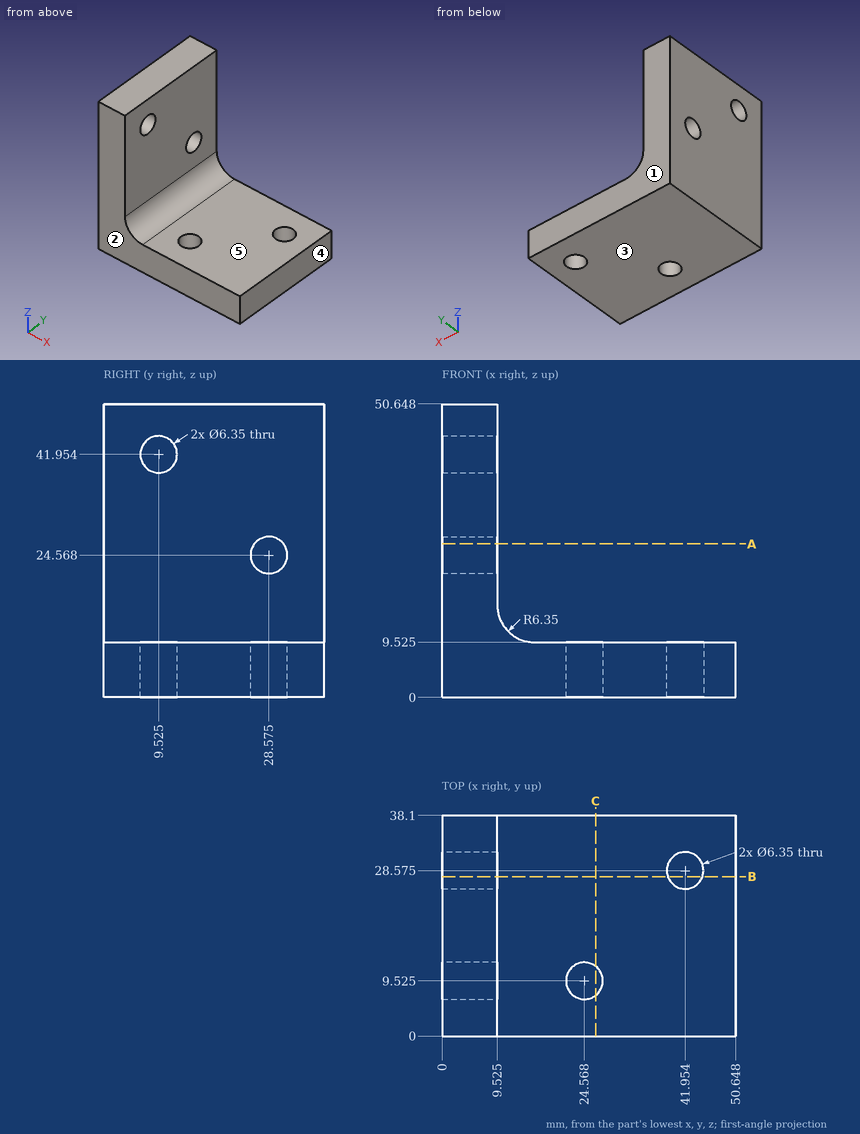
Source: three-view drawing plus pictorial views. Frame: mm from the lowest corner of the part. A direction names the side the tool comes from. Give positions to 0.01 mm unless a question says otherwise; leave off trailing zeros. Write each loop counter-clockwise with the first axis right and the second up, starting at its lowest first coordinate (ties: lowest second). Pieces come first, ordered by that corner, then holes. Notation, with made-up numbers: (-31.5, -10) - (-26.5, -10) arc R9 cw to (-26.5, 2) - close; hole circle Ø2 at (80, -12). An arc over 180 degrees is marked (long way). Write item = value, one per line. Start each with the question number.
1. Ray query, L1, parallel to X at y = 35.5, z = 43 (1 decimal); L2, parallel to Y at x = 5.5, z = 44.5 (1 decimal). Return the intervals inside material, ascending.
2. Section query B-B, the plane y = 27.5. Count the separate pieces of the cut face and the enclosed holes in it, then the cut area to 3 significant figures.
3. Section query A-A, the plane z = 26.5. Output: boundary loops of the cut face in (x, y) (1 decimal), then the cut area to 3 significant figures.
4. Access query for the marked faces 4 and 5. Directions: +Z, -Z, +X, -X, +Y, -Y. A direction counts if a zero-diameter tool reaches every point of the face in a straight line with its end or side. Return the directions, or none.
5. First-contact query: pin 1 Ø17.5 at (y, z) = (12, 40.5) entering from +X (3 decimals). Flat tip, straight axial feed; report the tip coordinate or a pass-through.
6. Section query C-C, the plane x = 26.5. Output: boundary loops of the cut face in (y, z) (1 decimal), then the cut area to 3 significant figures.
7. Mould query, pull axis Y, two halves, no side actions, for the marked faces 1, 2 and 3. Classes: released by +Y, released by -Y, zero draft, split by the parting line, or undercut.
Check sheet entries:
q1.L1 = 0 to 9.5
q1.L2 = 0 to 7.6, 11.4 to 38.1
q2.separate_pieces = 3
q2.enclosed_holes = 0
q2.area = 769 mm2
q3.outline = (0, 0) - (9.5, 0) - (9.5, 26.1) - (0, 26.1) - close; (0, 31.1) - (9.5, 31.1) - (9.5, 38.1) - (0, 38.1) - close
q3.area = 315 mm2
q4.face_4 = +Z, -Z, +X, +Y, -Y
q4.face_5 = +Z, +X, +Y, -Y
q5.pin_1 = 9.525
q6.outline = (0, 0) - (7, 0) - (7, 9.5) - (0, 9.5) - close; (12, 0) - (38.1, 0) - (38.1, 9.5) - (12, 9.5) - close
q6.area = 315 mm2
q7.face_1 = released by +Y
q7.face_2 = released by -Y
q7.face_3 = zero draft
